Can you work these out from the model? Positions are in its coordinate system, mm. A direction names the side the tool comes from. Round coordinates to 2 decimals unless told otherwise and drop trailing zeros. Write each loop counter-clockwise with the first axis right and the second up, starting at its lowest first coordinate (ties: lowest second). Pieces come first, ordered by that corner, then holes. Notation, with made-up numbers: M 36.5,-3.5 L 88.5,-3.5 A20 cw 88.5,8.5 Z; hole C 20.25,-1 d6. An arc over 180 degrees is marked long. Answer in a Markdown table with one row per item. Add a question column.
(1) If I drill on probe 1 along Z at (x, y) = (47, -1.5); probe 2 along Z at (x, y) = (129, -0.25); probe 3 along Y at (x, z) = (-89.5, 9.5), over which ranges is the centre line in solid material (lowest first)?
(2) Suppose I cut it at B-B, the plane x = -99. Write out the boundary of the cut face in (y, z) (3 decimals).
(3) For faces 5 (the face through (-2, 0, 0)), 6 (the face through (-2, -1, 0)), which set-ups out of +Z, -Z, +X, -X, +Y, -Y let a thin tool reach every point of the face, with its end or its side?
(4) If we mould it in two halves opening along Z, with no side actions, what happens to faces 1 (the face through (2, -7, 19.335)), 2 (the face through (2, -7, 20.335)), 3 (the face through (-2, -7, -19.335)), 4 (the face through (-2, -7, -20.335))? For each: released by +Z, released by -Z, zero draft, split by the parting line, or undercut.
(5) I'm going to push flat-ended pins straight in: pin 1 (2.5 mm diameter, centred on x = 129, z = 12, fed in from +Y); pin 2 (1.1 mm diameter, centred on x = -122, y = -0.5, fed in from -Z); pin 3 (0.5 mm diameter, centred on x = -128, y = -0.5, fed in from -Z); pin 4 (1.1 mm diameter, centred on x = -41, y = -0.5, fed in from +Z). Where does each tip first touch, or does it pass through?
(6) Suppose I cut it at A-A, the plane z = 0. Write out the boundary of the cut face in (x, y), then the cut area to 3 significant figures.
from build123d import *

# Parameters (mm, degrees)
SKETCH1_W               = 270
SKETCH1_H               = 37.4
BASE_FLANGE1_DEPTH      = 1
SKETCH4_R               = 4
CUT_EXTRUDE1_DEPTH      = 137.292663045
CUT_EXTRUDE2_DEPTH      = 1
EDGE_FLANGE1_DEPTH      = 250
EDGE_FLANGE1_BEND_DEPTH = 250
CUT_EXTRUDE3_REACH      = 139.14
SKETCH13_R              = 1.7
CUT_EXTRUDE4_DEPTH      = 142.591132844
BREAK_CORNER1_START     = -20.335
BREAK_CORNER1_DEPTH     = 40.67
BREAK_CORNER1_START_2   = -1
BREAK_CORNER1_2_DEPTH   = 1
CUT_EXTRUDE5_REACH      = 139.14
SKETCH16_R              = 1.7
CUT_EXTRUDE6_DEPTH      = 142.591132844
CUT_EXTRUDE7_DEPTH      = 1


# Read off the part's stored shape, not the designer's step: Break-Corner1
# Sheet-metal steps are written as plain solids
with BuildPart() as part:
    # Sketch1 → Base-Flange1 (new body)
    with BuildSketch(Plane(origin=(0, 0, 0), x_dir=(1, 0, 0), z_dir=(0, 1, 0))):
        Rectangle(SKETCH1_W, SKETCH1_H)
    extrude(amount=-BASE_FLANGE1_DEPTH)

    # Sketch4 → Cut-Extrude1 (cut, through all)
    with BuildSketch(Plane(origin=(0, 0, 0), x_dir=(1, 0, 0), z_dir=(0, 1, 0))):
        with Locations(Location((-40, 0, 0), (0, 0, 270))):
            Circle(SKETCH4_R)
        with Locations(Location((40, 0, 0), (0, 0, 90))):
            Circle(SKETCH4_R)
    extrude(amount=-CUT_EXTRUDE1_DEPTH, mode=Mode.SUBTRACT)

    # Sketch6 → Cut-Extrude2 (cut)
    with BuildSketch(Plane(origin=(0, 0, 0), x_dir=(1, 0, 0), z_dir=(0, 1, 0))):
        with BuildLine():
            Line((-45, 4), (-35, 4))
            ThreePointArc((-35, 4), (-31, 0), (-35, -4))
            Line((-35, -4), (-45, -4))
            ThreePointArc((-45, -4), (-49, 0), (-45, 4))
        make_face()
    extrude(amount=-CUT_EXTRUDE2_DEPTH, mode=Mode.SUBTRACT)

    # Edge-Flange1 section (across the edge) → Edge-Flange1 (add)
    with BuildSketch(Plane(origin=(125, -1, 19.335), x_dir=(0, 0, -1), z_dir=(-1, 0, 0))):
        with BuildLine():
            Line((-1, 0.635), (-1, 12))
            Line((-1, 12), (0, 12))
            Line((0, 12), (0, 0.635))
            ThreePointArc((0, 0.635), (0.185987194, 0.185987194), (0.635, 0))
            Line((0.635, 0), (0.635, -1))
            ThreePointArc((0.635, -1), (-0.521119587, -0.521119587), (-1, 0.635))
        make_face()
    extrude(amount=EDGE_FLANGE1_DEPTH)

    # Edge-Flange1 section 2 (across the edge) → Edge-Flange1 bend (add)
    with BuildSketch(Plane(origin=(-125, -1, -19.335), x_dir=(0, 0, 1), z_dir=(1, 0, 0))):
        with BuildLine():
            Line((-1, 0.635), (-1, 12))
            Line((-1, 12), (0, 12))
            Line((0, 12), (0, 0.635))
            ThreePointArc((0, 0.635), (0.185987194, 0.185987194), (0.635, 0))
            Line((0.635, 0), (0.635, -1))
            ThreePointArc((0.635, -1), (-0.521119587, -0.521119587), (-1, 0.635))
        make_face()
    extrude(amount=EDGE_FLANGE1_BEND_DEPTH)

    # Sketch13 → Cut-Extrude3 (cut, up to next)
    with BuildSketch(Plane(origin=(0, 0, 0), x_dir=(1, 0, 0), z_dir=(0, 1, 0)), mode=Mode.PRIVATE) as cut_extrude3_sk1:
        with Locations(Location((-129, 12, 0), (0, 0, 270))):
            Circle(SKETCH13_R)
    cut_extrude3_tool1 = extrude(cut_extrude3_sk1.sketch, amount=-CUT_EXTRUDE3_REACH, mode=Mode.PRIVATE) & part.part
    # Sketch13 → Cut-Extrude3 (cut, up to next)
    with BuildSketch(Plane(origin=(0, 0, 0), x_dir=(1, 0, 0), z_dir=(0, 1, 0)), mode=Mode.PRIVATE) as cut_extrude3_sk2:
        with Locations(Location((-129, -12, 0), (0, 0, 270))):
            Circle(SKETCH13_R)
    cut_extrude3_tool2 = extrude(cut_extrude3_sk2.sketch, amount=-CUT_EXTRUDE3_REACH, mode=Mode.PRIVATE) & part.part
    # Sketch13 → Cut-Extrude3 (cut, up to next)
    with BuildSketch(Plane(origin=(0, 0, 0), x_dir=(1, 0, 0), z_dir=(0, 1, 0)), mode=Mode.PRIVATE) as cut_extrude3_sk3:
        with Locations(Location((129, -12, 0), (0, 0, 270))):
            Circle(SKETCH13_R)
    cut_extrude3_tool3 = extrude(cut_extrude3_sk3.sketch, amount=-CUT_EXTRUDE3_REACH, mode=Mode.PRIVATE) & part.part
    # Sketch13 → Cut-Extrude3 (cut, up to next)
    with BuildSketch(Plane(origin=(0, 0, 0), x_dir=(1, 0, 0), z_dir=(0, 1, 0)), mode=Mode.PRIVATE) as cut_extrude3_sk4:
        with Locations(Location((129, 12, 0), (0, 0, 270))):
            Circle(SKETCH13_R)
    cut_extrude3_tool4 = extrude(cut_extrude3_sk4.sketch, amount=-CUT_EXTRUDE3_REACH, mode=Mode.PRIVATE) & part.part
    add(cut_extrude3_tool1.solids().sort_by_distance((-129, 0, -12))[0], mode=Mode.SUBTRACT)
    add(cut_extrude3_tool2.solids().sort_by_distance((-129, 0, 12))[0], mode=Mode.SUBTRACT)
    add(cut_extrude3_tool3.solids().sort_by_distance((129, 0, 12))[0], mode=Mode.SUBTRACT)
    add(cut_extrude3_tool4.solids().sort_by_distance((129, 0, -12))[0], mode=Mode.SUBTRACT)

    # Sketch14 → Cut-Extrude4 (cut, through all)
    with BuildSketch(Plane.XY.offset(20.335)):
        with BuildLine():
            Line((78, -5.6675), (101, -5.6675))
            ThreePointArc((101, -5.6675), (102.65, -7.3175), (101, -8.9675))
            Line((101, -8.9675), (78, -8.9675))
            ThreePointArc((78, -8.9675), (76.35, -7.3175), (78, -5.6675))
        make_face()
    extrude(amount=-CUT_EXTRUDE4_DEPTH, mode=Mode.SUBTRACT)

    # Break-Corner1 outline → Break-Corner1 (cut)
    with BuildSketch(Plane.XY.offset(BREAK_CORNER1_START)):
        with BuildLine():
            Line((-125, -13), (-122.5, -13))
            ThreePointArc((-122.5, -13), (-124.267766953, -12.267766953), (-125, -10.5))
            Line((-125, -10.5), (-125, -13))
        make_face()
        with BuildLine():
            ThreePointArc((125, -10.5), (124.267766953, -12.267766953), (122.5, -13))
            Line((122.5, -13), (125, -13))
            Line((125, -13), (125, -10.5))
        make_face()
    extrude(amount=BREAK_CORNER1_DEPTH, mode=Mode.SUBTRACT)

    # Break-Corner1 2 outline → Break-Corner1 2 (cut)
    with BuildSketch(Plane(origin=(0, 0, 0), x_dir=(1, 0, 0), z_dir=(0, 1, 0)).offset(BREAK_CORNER1_START_2)):
        with BuildLine():
            ThreePointArc((132.5, 18.7), (134.267766953, 17.967766953), (135, 16.2))
            Line((135, 16.2), (135, 18.7))
            Line((135, 18.7), (132.5, 18.7))
        make_face()
        with BuildLine():
            ThreePointArc((135, -16.2), (134.267766953, -17.967766953), (132.5, -18.7))
            Line((132.5, -18.7), (135, -18.7))
            Line((135, -18.7), (135, -16.2))
        make_face()
        with BuildLine():
            Line((-135, 18.7), (-135, 16.2))
            ThreePointArc((-135, 16.2), (-134.267766953, 17.967766953), (-132.5, 18.7))
            Line((-132.5, 18.7), (-135, 18.7))
        make_face()
        with BuildLine():
            ThreePointArc((-132.5, -18.7), (-134.267766953, -17.967766953), (-135, -16.2))
            Line((-135, -16.2), (-135, -18.7))
            Line((-135, -18.7), (-132.5, -18.7))
        make_face()
    extrude(amount=BREAK_CORNER1_2_DEPTH, mode=Mode.SUBTRACT)

    # Sketch15 → Cut-Extrude5 (cut, up to next)
    with BuildSketch(Plane(origin=(0, 0, 0), x_dir=(1, 0, 0), z_dir=(0, 1, 0)), mode=Mode.PRIVATE) as cut_extrude5_sk1:
        with BuildLine():
            Line((-6, -10.8), (6, -10.8))
            ThreePointArc((6, -10.8), (7.7, -12.5), (6, -14.2))
            Line((6, -14.2), (-6, -14.2))
            ThreePointArc((-6, -14.2), (-7.7, -12.5), (-6, -10.8))
        make_face()
    cut_extrude5_tool1 = extrude(cut_extrude5_sk1.sketch, amount=-CUT_EXTRUDE5_REACH, mode=Mode.PRIVATE) & part.part
    # Sketch15 → Cut-Extrude5 (cut, up to next)
    with BuildSketch(Plane(origin=(0, 0, 0), x_dir=(1, 0, 0), z_dir=(0, 1, 0)), mode=Mode.PRIVATE) as cut_extrude5_sk2:
        with BuildLine():
            Line((-6, 10.8), (6, 10.8))
            ThreePointArc((6, 10.8), (7.7, 12.5), (6, 14.2))
            Line((6, 14.2), (-6, 14.2))
            ThreePointArc((-6, 14.2), (-7.7, 12.5), (-6, 10.8))
        make_face()
    cut_extrude5_tool2 = extrude(cut_extrude5_sk2.sketch, amount=-CUT_EXTRUDE5_REACH, mode=Mode.PRIVATE) & part.part
    add(cut_extrude5_tool1.solids().sort_by_distance((0, 0, 12.5))[0], mode=Mode.SUBTRACT)
    add(cut_extrude5_tool2.solids().sort_by_distance((0, 0, -12.5))[0], mode=Mode.SUBTRACT)

    # Sketch16 → Cut-Extrude6 (cut, through all)
    with BuildSketch(Plane.XY.offset(20.335)):
        with Locations(Location((15, -7.3175, 0), (0, 0, 270))):
            Circle(SKETCH16_R)
        with Locations(Location((-15, -7.3175, 0), (0, 0, 270))):
            Circle(SKETCH16_R)
    extrude(amount=-CUT_EXTRUDE6_DEPTH, mode=Mode.SUBTRACT)

    # Sketch17 → Cut-Extrude7 (cut)
    with BuildSketch(Plane(origin=(0, 0, 0), x_dir=(1, 0, 0), z_dir=(0, 1, 0))):
        with BuildLine():
            Line((-129, -10.3), (-119, -10.3))
            ThreePointArc((-119, -10.3), (-117.3, -12), (-119, -13.7))
            Line((-119, -13.7), (-129, -13.7))
            ThreePointArc((-129, -13.7), (-130.7, -12), (-129, -10.3))
        make_face()
        with BuildLine():
            Line((-129, 13.7), (-119, 13.7))
            ThreePointArc((-119, 13.7), (-117.3, 12), (-119, 10.3))
            Line((-119, 10.3), (-129, 10.3))
            ThreePointArc((-129, 10.3), (-130.7, 12), (-129, 13.7))
        make_face()
    extrude(amount=-CUT_EXTRUDE7_DEPTH, mode=Mode.SUBTRACT)


solid = part.part
Calculated:
| question | item | result |
|---|---|---|
| 1 | probe 1 | -20.33 to -19.32, 19.32 to 20.33 |
| 1 | probe 2 | -18.7 to -13.7, -10.3 to 10.3, 13.7 to 18.7 |
| 1 | probe 3 | -1 to 0 |
| 2 | outline | M -13,-20.335 L -1.635,-20.335 A1.635 ccw 0,-18.7 L 0,18.7 A1.635 ccw -1.635,20.335 L -13,20.335 L -13,19.335 L -1.635,19.335 A0.635 cw -1,18.7 L -1,-18.7 A0.635 cw -1.635,-19.335 L -13,-19.335 Z |
| 3 | face 5 | +Z, -Z, +X, -X, +Y |
| 3 | face 6 | +X, -X, -Y |
| 4 | face 1 | undercut |
| 4 | face 2 | released by +Z |
| 4 | face 3 | undercut |
| 4 | face 4 | released by -Z |
| 5 | pin 1 | through |
| 5 | pin 2 | z = -20.23 |
| 5 | pin 3 | z = -18.7 |
| 5 | pin 4 | z = 20.23 |
| 6 | outline | M -135,-1 L -49,-1 L -49,0 L -135,0 Z; M -31,-1 L 36,-1 L 36,0 L -31,0 Z; M 44,-1 L 135,-1 L 135,0 L 44,0 Z |
| 6 | area | 244 mm² |
